The listing builds one solid part. Answer for the finished solid, in the listing's coordinates (mm). Face numbers are marked on the shaded views. A direction names the side the tool comes from. Round coordinates to 2 decimals unless told otherwise and drop trailing zeros. Write each loop counter-clockwise with the first axis right and the second up, starting at its lowest first coordinate (ties: lowest second). Pieces come first, ordered by that corner, then holes. Notation, with made-up numbers: (13.5, -19.5) - (50.5, -19.5) arc R16 cw to (50.5, -9.5) - close; hole circle Ø2 at (11, 37). An arc over 180 degrees is marked (long way). Answer in a Markdown table with one row per item.
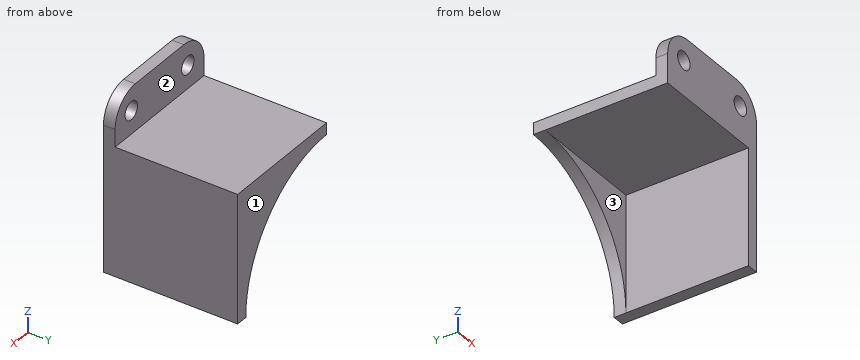
from build123d import *

# Parameters (mm, degrees)
CYLINDER001_R          = 20
CYLINDER001_DEPTH      = 25
CYLINDER001_ROLL_ANGLE = -90
CYLINDER002_R          = 1.55
CYLINDER002_DEPTH      = 10
CYLINDER002_ROLL_ANGLE = -90
CYLINDER_R             = 1.55
CYLINDER_DEPTH         = 10
CYLINDER_ROLL_ANGLE    = -90
BOX003_W               = 10
BOX003_H               = 6
BOX003_DEPTH           = 31
BOX001_W               = 20
BOX001_H               = 21
BOX001_DEPTH           = 20
BOX_W                  = 22
BOX_H                  = 23
BOX_DEPTH              = 22
BOX002_W               = 30
BOX002_H               = 2
BOX002_DEPTH           = 30
FILLET_R               = 5
FILLET001_R            = 5


with BuildPart() as cilindro001:
    # Cylinder001 → Cylinder001 (new body)
    with BuildSketch(Plane.XY):
        Circle(CYLINDER001_R)
    extrude(amount=CYLINDER001_DEPTH)


with BuildPart() as cilindro001_1:
    # Cylinder001 roll: moved
    add(cilindro001.part.rotate(Axis((0, 0, 0), (1, 0, 0)), CYLINDER001_ROLL_ANGLE))


with BuildPart() as cilindro001_2:
    # Cylinder001 placement: moved
    add(cilindro001_1.part)


with BuildPart() as cilindro002:
    # Cylinder002 → Cylinder002 (new body)
    with BuildSketch(Plane.XY):
        Circle(CYLINDER002_R)
    extrude(amount=CYLINDER002_DEPTH)


with BuildPart() as cilindro002_1:
    # Cylinder002 roll: moved
    add(cilindro002.part.rotate(Axis((0, 0, 0), (1, 0, 0)), CYLINDER002_ROLL_ANGLE))


with BuildPart() as cilindro002_2:
    # Cylinder002 placement: moved
    add(cilindro002_1.part.moved(Location((4, -2, 26))))


with BuildPart() as cilindro:
    # Cylinder → Cylinder (new body)
    with BuildSketch(Plane.XY):
        Circle(CYLINDER_R)
    extrude(amount=CYLINDER_DEPTH)


with BuildPart() as cilindro_1:
    # Cylinder roll: moved
    add(cilindro.part.rotate(Axis((0, 0, 0), (1, 0, 0)), CYLINDER_ROLL_ANGLE))


with BuildPart() as cilindro_2:
    # Cylinder placement: moved
    add(cilindro_1.part.moved(Location((18, -2, 26))))


with BuildPart() as cubo003:
    # Box003 → Box003 (new body)
    with BuildSketch(Plane(origin=(22, 0, 0), x_dir=(1, 0, 0), z_dir=(0, 0, 1))):
        with Locations((5, 3)):
            Rectangle(BOX003_W, BOX003_H)
    extrude(amount=BOX003_DEPTH)


with BuildPart() as cubo001:
    # Box001 → Box001 (new body)
    with BuildSketch(Plane.XY):
        with Locations((10, 10.5)):
            Rectangle(BOX001_W, BOX001_H)
    extrude(amount=BOX001_DEPTH)


with BuildPart() as cubo:
    # Box → Box (new body)
    with BuildSketch(Plane.XY):
        with Locations((11, 11.5)):
            Rectangle(BOX_W, BOX_H)
    extrude(amount=BOX_DEPTH)


with BuildPart() as fillet001:
    # Box002 → Box002 (new body)
    with BuildSketch(Plane.XY):
        with Locations((15, 1)):
            Rectangle(BOX002_W, BOX002_H)
    extrude(amount=BOX002_DEPTH)

    # Fusion: union Cubo
    add(cubo.part)

    # Cut: cut Cubo001
    add(cubo001.part, mode=Mode.SUBTRACT)

    # Cut001: cut Cubo003
    add(cubo003.part, mode=Mode.SUBTRACT)

    # Cut002: cut Cilindro
    add(cilindro_2.part, mode=Mode.SUBTRACT)

    # Cut003: cut Cilindro002
    add(cilindro002_2.part, mode=Mode.SUBTRACT)

    # Cut004: cut Cilindro001
    add(cilindro001_2.part, mode=Mode.SUBTRACT)

    # Fillet
    fillet_edges = [fillet001.edges().sort_by_distance(p)[0] for p in [
        (0, 1, 30),
    ]]
    fillet(fillet_edges, radius=FILLET_R)

    # Fillet001
    fillet001_edges = [fillet001.edges().sort_by_distance(p)[0] for p in [
        (22, 1, 30),
    ]]
    fillet(fillet001_edges, radius=FILLET001_R)


solid = fillet001.part
(1) Section D-D (z = 6.5) is taken. Give the vertices of the cut face in (x, y).
Checked values:
| item | result |
|---|---|
| outline | (18.91, 21) - (20, 21) - (20, 0) - (22, 0) - (22, 23) - (18.91, 23) - close |
(2) For the marked faces 1, 2 and 3, determine the directions among +Z, -Z, +X, -X, +Y, -Y from which every point of the face is accessible in a straight line to the end or side of a thin tool.
Checked values:
| item | result |
|---|---|
| face 1 | +Z, -Z, +X, -X, +Y |
| face 2 | +Z, +X, -X, +Y |
| face 3 | -Z, -X, -Y |
(3) Find the intervals of material crossed by line 1 (X direction, y = 9.75, z = 7.25); line 2 (Y direction, x = 12.75, z = 23.75), in increasing order.
Checked values:
| item | result |
|---|---|
| line 1 | x = 20 to 22 |
| line 2 | y = 0 to 2 |
(4) Section B-B (z = 26) is taken. Give the vertices of the cut face in (x, y), and give its area (3 significant figures).
Checked values:
| item | result |
|---|---|
| outline | (0.1, 0) - (2.45, 0) - (2.45, 2) - (0.1, 2) - close; (5.55, 0) - (16.45, 0) - (16.45, 2) - (5.55, 2) - close; (19.55, 0) - (21.9, 0) - (21.9, 2) - (19.55, 2) - close |
| area | 31.2 mm2 |
(5) Section A-A (x = 4) is taken. Give the vertices of the cut face in (y, z), and give its area (3 significant figures).
Checked values:
| item | result |
|---|---|
| outline | (0, 20) - (21, 20) - (21, 19.6) - (23, 19.6) - (23, 22) - (2, 22) - (2, 24.45) - (0, 24.45) - close; (0, 27.55) - (2, 27.55) - (2, 29.9) - (0, 29.9) - close |
| area | 56.4 mm2 |
(6) Section C-C (y = 20) is taken. Give the vertices of the cut face in (x, z).
Checked values:
| item | result |
|---|---|
| outline | (0, 20) - (20, 20) - (20, 0) - (22, 0) - (22, 22) - (0, 22) - close |
(7) Flat-ended cylindrical pins translate along their axes: pin 1 (6 mm diameter, centred on y = 5.5, z = 7, fed in from -X); pin 2 (8 mm diameter, centred on x = 11.5, y = 8, fed in from +Z); pin 3 (4 mm diameter, centred on x = 5, y = 16, fed in from -Z). Find the tip coordinate at first contact, or state that the pin passes through.
Checked values:
| item | result |
|---|---|
| pin 1 | stops at x = 20 |
| pin 2 | stops at z = 22 |
| pin 3 | stops at z = 20 |
